Autodesk Inventor part; units mm, degrees
ref_plane "YZ Plane" through (0, 0, 0) normal (1, 0, 0) x (0, 1, 0)
ref_plane "XZ Plane" through (0, 0, 0) normal (0, 1, 0) x (-1, 0, 0)
ref_plane "XY Plane" through (0, 0, 0) normal (0, 0, 1) x (1, 0, 0)
sketch "Sketch1" plane through (0, 0, 0) normal (0, 0, 1) x (1, 0, 0)
  line L0 (-41.5, 50) -> (41.5, 50)
  line L1 (41.5, 50) -> (41.5, -50)
  line L2 (41.5, -50) -> (-41.5, -50)
  line L3 (-41.5, -50) -> (-41.5, 50)
  line L4 (31.5, 40) -> (-31.5, 40)
  line L5 (-31.5, 40) -> (-31.5, -40)
  line L6 (-31.5, -40) -> (31.5, -40)
  line L7 (31.5, -40) -> (31.5, 40)
  line L8 (-41.5, -45) -> (41.5, -45) construction
  line L9 (0, 71.7466) -> (0, -78.0681) construction
  line L10 (-60.2597, 0) -> (74.2823, 0) construction
  line L11 (-36.5, 50) -> (-36.5, -50) construction
  circle A0 centre (-36.5, -27) radius 2.25
  line L12 (-41.5, 45) -> (41.5, 45) construction
  circle A1 centre (-36.5, 45) radius 2.25
  circle A2 centre (-36.5, -45) radius 2.25
  circle A3 centre (-36.5, 27) radius 2.25
  circle A4 centre (-25, -45) radius 2.25
  circle A5 centre (25, -45) radius 2.25
  line L13 (30, 50) -> (30, -50) construction
  line L14 (-30, 50) -> (-30, -50) construction
  line L15 (-31, -38) -> (31, -38)
  line L16 (31, -38) -> (31, -52)
  line L17 (31, -52) -> (-31, -52)
  line L18 (-31, -52) -> (-31, -38)
  line L19 (-31.5, -40) -> (-16.5, -40)
  line L20 (-16.5, -40) -> (-16.5, -20)
  line L21 (-16.5, -20) -> (-31.5, -20)
  line L22 (-31.5, -20) -> (-31.5, -40)
  line L23 (-26.5, -26) -> (-21.5, -26) construction
  line L24 (-26.5, -27.5) -> (-21.5, -27.5)
  line L25 (-21.5, -24.5) -> (-26.5, -24.5)
  arc A6 (-26.5, -24.5) -> (-26.5, -27.5) centre (-26.5, -26) ccw
  arc A7 (-21.5, -27.5) -> (-21.5, -24.5) centre (-21.5, -26) ccw
  line L26 (-26.5, -34) -> (-21.5, -34) construction
  line L27 (-26.5, -35.5) -> (-21.5, -35.5)
  line L28 (-21.5, -32.5) -> (-26.5, -32.5)
  arc A8 (-26.5, -32.5) -> (-26.5, -35.5) centre (-26.5, -34) ccw
  arc A9 (-21.5, -35.5) -> (-21.5, -32.5) centre (-21.5, -34) ccw
  point P0 (0, 0)
  point P1 (0, 50)
  point P2 (41.5, 0)
  point P3 (0, 45)
  point P4 (-24, -26)
  point P5 (-24, -20)
  point P6 (-16.5, -30)
  point P7 (-24, -34)
  dimension "d0" = 83
  dimension "d1" = 100
  dimension "d5" = 5
  dimension "d6" = 5
  dimension "d9" = 5
  dimension "d12" = 4.5
  dimension "d17" = 5
  dimension "d41" = 4.5
  dimension "d42" = 4.5
  dimension "d87" = 4.5
  dimension "d89" = 4.5
  dimension "d90" = 4.5
  dimension "d91" = 30
  dimension "d92" = 30
  dimension "d93" = 5
  dimension "d94" = 5
  dimension "d97" = 1
  dimension "d98" = 2
  dimension "d99" = 2
  dimension "d100" = 1
  dimension "d103" = 15
  dimension "d104" = 20
  dimension "d105" = 5
  dimension "d106" = 3
  dimension "d109" = 5
  dimension "d110" = 3
  dimension "d112" = 6
  dimension "d113" = 6
  dimension "d141" = 27
  dimension "d142" = 27
sketch "Sketch4" plane through (0, 0, 0) normal (0, 0, 1) x (1, 0, 0)
  circle A0 centre (-36.5, 27) radius 2.25
  circle A1 centre (-36.5, -27) radius 2.25
  line L0 (-31.5, 40) -> (-31.5, -40)
  line L1 (-41.5, -50) -> (-41.5, 50)
  line L2 (-41.5, -32.25) -> (-31.5, -32.25)
  line L3 (-31.5, -32.25) -> (-31.5, 32.25)
  line L4 (-31.5, 32.25) -> (-41.5, 32.25)
  line L5 (-41.5, 32.25) -> (-41.5, -32.25)
  line L6 (31.5, -40) -> (31.5, 40)
  line L7 (41.5, 50) -> (41.5, -50)
  line L8 (31.5, -18) -> (31.5, 0)
  line L9 (-31.5, 0) -> (-31.5, -18)
  line L10 (-16.5, -20) -> (-31.5, -20)
  line L11 (-31.5, -40) -> (31.5, -40)
  line L12 (-16.5, -40) -> (-16.5, -20)
  line L13 (-31.5, 14.5) -> (0, 14.5)
  line L14 (0, 14.5) -> (0, 6)
  line L15 (0, 6) -> (-31.5, 6)
  line L16 (-31.5, 6) -> (-31.5, 14.5)
  circle A2 centre (-9, 10.25) radius 1.5
  line L17 (0, 10.25) -> (-31.5, 10.25) construction
  circle A3 centre (-20, 10.25) radius 2.25
  line L18 (0, 28.3973) -> (0, -18) construction
  point P0 (0, 0)
  dimension "d116" = 3
  dimension "d117" = 3
  dimension "d151" = 8.5
  dimension "d152" = 3
  dimension "d153" = 9
  dimension "d154" = 22
  dimension "d155" = 4.5
  dimension "d156" = 20
extrude "Extrusion11" add sketch "Sketch4" along normal blind 1.5 contours L0 L2 L1 L4 | L13 L14 L15 L0
mirror "Mirror10" about plane through (0, 0, 0) normal (1, 0, 0) of "Extrusion11"
equation "\"d12\" = screw"
equation "\"d41\" = screw"
equation "\"d42\" = screw"
equation "\"d87\" = screw"
equation "\"d89\" = screw"
equation "\"d90\" = screw"
properties part number "Side" material "PC/ABS Plastic"
Geometry: final body of the model. Coordinates: model frame, mm. Round coordinates to 2 decimals unless told otherwise and drop trailing zeros. Write each loop counter-clockwise with the first axis right and the second up, starting at its lowest first coordinate (ties: lowest second). Pieces come first, ordered by that corner, then holes. Notation, with made-up numbers: (-36, 81) -> (18, 81) arc R31 ccw to (18, 114) -> close; hole circle Ø6 at (-1, -20.5). An arc over 180 degrees is marked (long way). Return JSON: item names as keys, results as strings.
Q1. First-contact query: pin 1 Ø2.5 at (x, y) = (9, 10.25) entering from -Z. Flat tip, straight axial feed; report the tip coordinate or a pass-through.
From the geometry:
{"pin 1": "through"}
Q2. Section D-D on x = 36.5. Return the cut outline in (y, z).
From the geometry:
{"outline": "(-32.25, 0) -> (-29.25, 0) -> (-29.25, 1.5) -> (-32.25, 1.5) -> close; (-24.75, 0) -> (24.75, 0) -> (24.75, 1.5) -> (-24.75, 1.5) -> close; (29.25, 0) -> (32.25, 0) -> (32.25, 1.5) -> (29.25, 1.5) -> close"}
Q3. Section B-B on x = -9. Return the cut outline in (y, z), and give its area (3 significant figures).
From the geometry:
{"outline": "(6, 0) -> (8.75, 0) -> (8.75, 1.5) -> (6, 1.5) -> close; (11.75, 0) -> (14.5, 0) -> (14.5, 1.5) -> (11.75, 1.5) -> close", "area": "8.25 mm2"}
Q4. Ray query, line 1 (Y direction, x = -36.5, z = 0.75); line 2 (X direction, y = -1.5, z = 0.6); line 3 (Y direction, x = 9, z = 1). Return the intervals inside material, ascending.
From the geometry:
{"line 1": "-32.25 to -29.25, -24.75 to 24.75, 29.25 to 32.25", "line 2": "-41.5 to -31.5, 31.5 to 41.5", "line 3": "6 to 8.75, 11.75 to 14.5"}
Q5. Section A-A on y = -27. Return the cut outline in (x, z).
From the geometry:
{"outline": "(-41.5, 0) -> (-38.75, 0) -> (-38.75, 1.5) -> (-41.5, 1.5) -> close; (-34.25, 0) -> (-31.5, 0) -> (-31.5, 1.5) -> (-34.25, 1.5) -> close; (31.5, 0) -> (34.25, 0) -> (34.25, 1.5) -> (31.5, 1.5) -> close; (38.75, 0) -> (41.5, 0) -> (41.5, 1.5) -> (38.75, 1.5) -> close"}
Q6. Section C-C on z = 0.45. Give the number of separate pieces and of enclosed holes in the cut face, and give its area (3 significant figures).
From the geometry:
{"separate pieces": "1", "enclosed holes": "8", "area": "1,720 mm2"}
Q7. Mould query, pull axis X, two halves, no side actions, for faces 1 (the cylindrical face through (-35.462, 28.996, 0.74)), 2 (the flat face through (0, 7, 0)), 3 (the cylindrical face through (35.462, -28.996, 0.74)). Classes: +X half, -X half, draft (parallel to the pull), parting line (faces both ways), or undercut.
From the geometry:
{"face 1": "undercut", "face 2": "draft", "face 3": "undercut"}
